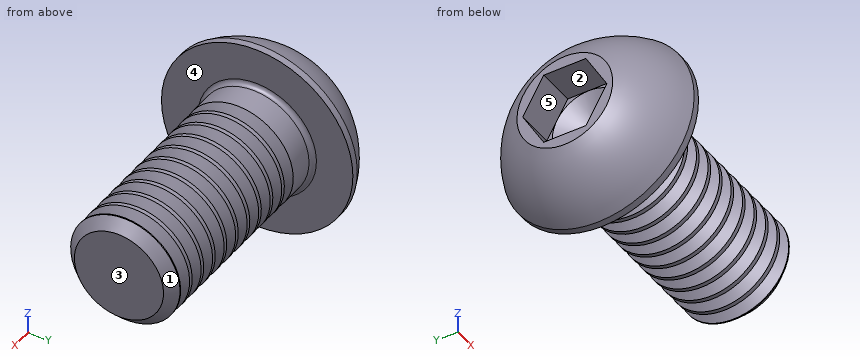
```python
from build123d import *

# Parameters (mm, degrees)
FILLET1_R       = 0.25
HEX_2_DEPTH     = 2.08
THDSCHPAT_COUNT = 10
THDSCHPAT_PITCH = 1


with BuildPart() as part:
    # BodySke → BaseBody (revolve)
    with BuildSketch(Plane.XY, mode=Mode.PRIVATE) as basebody_sk:
        with BuildLine():
            Line((15.3, 0), (15.3, 2.4455))
            Line((15.3, 2.4455), (14.7455, 3))
            Line((14.7455, 3), (3.3, 3))
            Line((3.3, 3), (3.3, 5.25))
            Line((3.3, 5.25), (2.92, 5.25))
            ThreePointArc((2.92, 5.25), (1.224500646, 4.199464996), (0, 2.625))
            Line((0, 2.625), (0, 0))
            Line((0, 0), (15.3, 0))
        make_face()
    revolve(basebody_sk.sketch.rotate(Axis((0, 0, 0), (1, 0, 0)), 90), axis=Axis((0, 0, 0), (1, 0, 0)))

    # Fillet1
    fillet1_edges = [part.edges().sort_by_distance(p)[0] for p in [
        (3.3, 0, -3),
    ]]
    fillet(fillet1_edges, radius=FILLET1_R)

    # Sketch2 → PreBroach (revolve, cut)
    with BuildSketch(Plane.XY, mode=Mode.PRIVATE) as prebroach_sk:
        Polygon((0, 2), (2.08, 2), (3.234700538, 0), (0, 0), align=None)
    revolve(prebroach_sk.sketch.rotate(Axis((0, 0, 0), (1, 0, 0)), 90), axis=Axis((0, 0, 0), (1, 0, 0)), mode=Mode.SUBTRACT)

    # Sketch3 → Hex 2 (cut)
    with BuildSketch(Plane(origin=(0, 0, 0), x_dir=(0, 0, -1), z_dir=(1, 0, 0))):
        Polygon((-2, -1.154700538), (-2, 1.154700538), (0, 2.309401077), (2, 1.154700538), (2, -1.154700538), (0, -2.309401077), align=None)
    extrude(amount=HEX_2_DEPTH, mode=Mode.SUBTRACT)

    # ThdSchSke → ThreadSchematic (revolve, cut)
    with BuildSketch(Plane.XY, mode=Mode.PRIVATE) as threadschematic_sk:
        Polygon((5.3, -2.4455), (4.91173492, -3), (4.91173492, -3.75), (5.68826508, -3.75), (5.68826508, -3), align=None)
    threadschematic = revolve(threadschematic_sk.sketch.rotate(Axis((-3.175, 0, 0), (1, 0, 0)), 270), axis=Axis((-3.175, 0, 0), (1, 0, 0)), mode=Mode.SUBTRACT)

    # ThdSchPat: ThreadSchematic ×10
    with Locations(*[(i * THDSCHPAT_PITCH, 0, 0) for i in range(1, THDSCHPAT_COUNT)]):
        add(threadschematic, mode=Mode.SUBTRACT)


solid = part.part
```
For this review, take the finished solid that the model builds, in its own axes (mm). Face numbers are marked on the shaded views. A direction names the side the tool comes from. Round coordinates to 2 decimals unless told otherwise and drop trailing zeros. Write each loop counter-clockwise with the first axis right and the second up, starting at its lowest first coordinate (ties: lowest second). Pieces come first, ordered by that corner, then holes. Notation, with made-up numbers: M 31.5,62.25 L 53.5,62.25 A23 ccw 53.5,93.25 Z; hole C 27,17.5 d11. An arc over 180 degrees is marked long. One line per item, written item: value. Start each with the question number.
(1) The part is to be moulded in two halves that separate along Y. For the marked faces 1, 2 and 3, say which applies: released by +Y, released by -Y, zero draft, split by the parting line, or undercut.
(2) Insertion check: pin 1 (0.5 mm diameter, centred on y = -0.5, z = 1.5, fed in from -X); pin 2 (1.5 mm diameter, centred on x = 12.5, z = 4, fed in from -Y); pin 3 (2.5 mm diameter, centred on x = 0.5, y = 0.5, fed in from +Z); pin 4 (1.5 mm diameter, centred on x = 10, z = 3, fed in from +Y). Each pin has a flat end and moves straight along its axis. Give the tip position at first contact, or say it passes through.
(3) We need section B-B (y = -3.75). Give the boundary of the cut face in (x, z), and give its area (3 significant figures).
(4) We need section A-A (z = 4.5). Give the boundary of the cut face in (x, y), and give its area (3 significant figures).
(5) Wall thickness on line 1 (Y direction, x = 0.75, z = 0.5); line 2 (Y direction, x = 3, z = -0.25); line 3 (Y direction, x = 13.25, z = 1): over which ranges is each line inside the solid? List them lowest first.
(6) Machinability: for the marked faces 4 and 5, which of the approach directions +Z, -Z, +X, -X, +Y, -Y give a long, thin tool a straight path to every point of the face, cutting with its end or side? Answer none if there is none.
Result:
1. face 1: split by the parting line
1. face 2: undercut
1. face 3: zero draft
2. pin 1: x = 2.18
2. pin 2: through
2. pin 3: z = 4.6
2. pin 4: y = 1.98
3. outline: M 2.92,-3.67 L 3.3,-3.67 L 3.3,3.67 L 2.92,3.67 A4.22 ccw Z
3. area: 14.0 mm²
4. outline: M 2.92,-2.7 L 3.3,-2.7 L 3.3,2.7 L 2.92,2.7 A3.41 ccw Z
4. area: 7.08 mm²
5. line 1: -3.68 to -2.02, 2.02 to 3.68
5. line 2: -5.24 to -0.32, 0.32 to 5.24
5. line 3: -2.31 to 2.31
6. face 4: +X
6. face 5: -X
